Read the model definition and answer for the solid it produces. Units are mm, in the model's axes. Give positions to 0.01 mm unless a question says otherwise; leave off trailing zeros. Order: outer loops, then holes, each group sorted by start corner. A loop starts at its lowest first (then second) coordinate and runs counter-clockwise, first axis right, second up. Notation, with made-up numbers: (33.5, -35.5) -> (77.5, -35.5) arc R21 ccw to (77.5, -27.5) -> close; hole circle Ø10 at (30.25, -13). An arc over 180 degrees is marked (long way). Answer as CSV lines item,"result". Start each with the question number.
1) Straight lines are drawn through the part: L1, parallel to Y at x = 5.5, z = 0.6; L2, parallel to X at y = -6.5, z = 0.8; L3, parallel to Y at x = -12, z = -0.85. For each, find the intervals that lie inside material, in ascending order. Write a range as from..to.
2) Find section B-B (y = -24). Determine the outline of the cut face in (x, z), and give its area (3 significant figures).
3) Find section D-D (y = -3). Determine the outline of the cut face in (x, z), and give its area (3 significant figures).
4) Find section C-C (z = -1.1). State how many separate pieces and enclosed holes the cut face has, and give its area (3 significant figures).
5) Flat-ended cylindrical pins translate along their axes: pin 1 Ø1.5 at (x, z) = (18, 1) entering from -Y; pin 2 Ø6 at (x, y) = (-18.5, -17) entering from -Z. Find the tip coordinate at first contact, or state that the pin passes through.
6) Find section A-A (x = 3). Determine the outline of the cut face in (y, z).
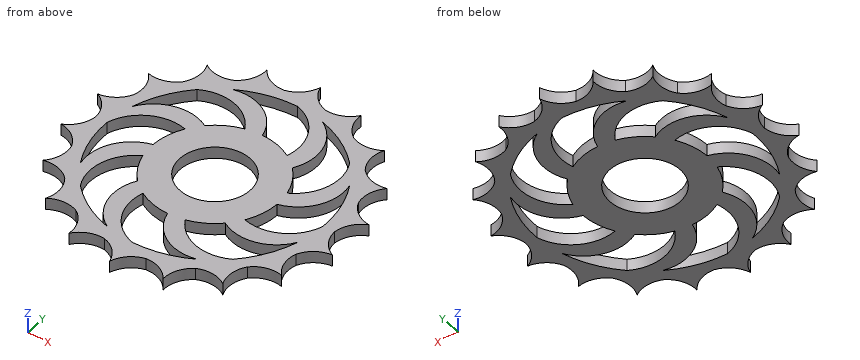
```python
from build123d import *

# Parameters (mm, degrees)
SALIENTE_EXTRUIR1_DEPTH = 1.5875
CROQUIS2_R              = 9.525
CORTAR_EXTRUIR1_DEPTH   = 4.175


with BuildPart() as part:
    # Croquis1 → Saliente-Extruir1 (new body, symmetric)
    with BuildSketch(Plane.XY):
        with BuildLine():
            ThreePointArc((0, 38.1), (-2.105039418, 34.526506764), (-5.733862827, 32.518352004))
            ThreePointArc((-5.733862827, 32.518352004), (-9.830670784, 33.164269511), (-13.030967461, 35.802288852))
            ThreePointArc((-13.030967461, 35.802288852), (-13.7868508, 31.724337744), (-16.51, 28.596158833))
            ThreePointArc((-16.51, 28.596158833), (-20.580657004, 27.801931903), (-24.490207929, 29.186293283))
            ThreePointArc((-24.490207929, 29.186293283), (-23.805764502, 25.09574539), (-25.294787512, 21.224846872))
            ThreePointArc((-25.294787512, 21.224846872), (-28.848312252, 19.086270994), (-32.995567884, 19.05))
            ThreePointArc((-32.995567884, 19.05), (-30.95335167, 15.440235769), (-31.028650338, 11.293505133))
            ThreePointArc((-31.028650338, 11.293505133), (-33.636435286, 8.06852412), (-37.52117539, 6.615995569))
            ThreePointArc((-37.52117539, 6.615995569), (-34.367507804, 3.922405841), (-33.02, 0))
            ThreePointArc((-33.02, 0), (-34.367507804, -3.922405841), (-37.52117539, -6.615995569))
            ThreePointArc((-37.52117539, -6.615995569), (-33.636435286, -8.06852412), (-31.028650338, -11.293505133))
            ThreePointArc((-31.028650338, -11.293505133), (-30.95335167, -15.440235769), (-32.995567884, -19.05))
            ThreePointArc((-32.995567884, -19.05), (-28.848312252, -19.086270994), (-25.294787512, -21.224846872))
            ThreePointArc((-25.294787512, -21.224846872), (-23.805764502, -25.09574539), (-24.490207929, -29.186293283))
            ThreePointArc((-24.490207929, -29.186293283), (-20.580657004, -27.801931903), (-16.51, -28.596158833))
            ThreePointArc((-16.51, -28.596158833), (-13.7868508, -31.724337744), (-13.030967461, -35.802288852))
            ThreePointArc((-13.030967461, -35.802288852), (-9.830670784, -33.164269511), (-5.733862827, -32.518352004))
            ThreePointArc((-5.733862827, -32.518352004), (-2.105039418, -34.526506764), (0, -38.1))
            ThreePointArc((0, -38.1), (2.105039418, -34.526506764), (5.733862827, -32.518352004))
            ThreePointArc((5.733862827, -32.518352004), (9.830670784, -33.164269511), (13.030967461, -35.802288852))
            ThreePointArc((13.030967461, -35.802288852), (13.7868508, -31.724337744), (16.51, -28.596158833))
            ThreePointArc((16.51, -28.596158833), (20.580657004, -27.801931903), (24.490207929, -29.186293283))
            ThreePointArc((24.490207929, -29.186293283), (23.805764502, -25.09574539), (25.294787512, -21.224846872))
            ThreePointArc((25.294787512, -21.224846872), (28.848312252, -19.086270994), (32.995567884, -19.05))
            ThreePointArc((32.995567884, -19.05), (30.95335167, -15.440235769), (31.028650338, -11.293505133))
            ThreePointArc((31.028650338, -11.293505133), (33.636435286, -8.06852412), (37.52117539, -6.615995569))
            ThreePointArc((37.52117539, -6.615995569), (34.367507804, -3.922405841), (33.02, 0))
            ThreePointArc((33.02, 0), (34.367507804, 3.922405841), (37.52117539, 6.615995569))
            ThreePointArc((37.52117539, 6.615995569), (33.636435286, 8.06852412), (31.028650338, 11.293505133))
            ThreePointArc((31.028650338, 11.293505133), (30.95335167, 15.440235769), (32.995567884, 19.05))
            ThreePointArc((32.995567884, 19.05), (28.848312252, 19.086270994), (25.294787512, 21.224846872))
            ThreePointArc((25.294787512, 21.224846872), (23.805764502, 25.09574539), (24.490207929, 29.186293283))
            ThreePointArc((24.490207929, 29.186293283), (20.580657004, 27.801931903), (16.51, 28.596158833))
            ThreePointArc((16.51, 28.596158833), (13.7868508, 31.724337744), (13.030967461, 35.802288852))
            ThreePointArc((13.030967461, 35.802288852), (9.830670784, 33.164269511), (5.733862827, 32.518352004))
            ThreePointArc((5.733862827, 32.518352004), (2.105039418, 34.526506764), (0, 38.1))
        make_face()
    extrude(amount=SALIENTE_EXTRUIR1_DEPTH, both=True)

    # Croquis2 → Cortar-Extruir1 (cut, through all)
    with BuildSketch(Plane.XY.offset(1.5875)):
        Circle(CROQUIS2_R)
        with BuildLine():
            ThreePointArc((8.5725, 14.848005548), (4.437452528, 16.560798292), (0, 17.145))
            ThreePointArc((0, 17.145), (-5.659104508, 24.58631503), (-14.9225, 25.846528176))
            ThreePointArc((-14.9225, 25.846528176), (-7.724454401, 28.828056286), (0, 29.845))
            ThreePointArc((0, 29.845), (7.392229248, 24.121925656), (8.5725, 14.848005548))
        make_face()
        with BuildLine():
            ThreePointArc((21.103601885, 21.103601885), (14.9225, 25.846528176), (7.724454401, 28.828056286))
            ThreePointArc((7.724454401, 28.828056286), (13.383558909, 21.386741255), (12.123345763, 12.123345763))
            ThreePointArc((12.123345763, 12.123345763), (14.848005548, 8.5725), (16.560798292, 4.437452528))
            ThreePointArc((16.560798292, 4.437452528), (22.283872636, 11.829681777), (21.103601885, 21.103601885))
        make_face()
        with BuildLine():
            ThreePointArc((29.845, 0), (28.828056286, 7.724454401), (25.846528176, 14.9225))
            ThreePointArc((25.846528176, 14.9225), (24.58631503, 5.659104508), (17.145, 0))
            ThreePointArc((17.145, 0), (16.560798292, -4.437452528), (14.848005548, -8.5725))
            ThreePointArc((14.848005548, -8.5725), (24.121925656, -7.392229248), (29.845, 0))
        make_face()
        with BuildLine():
            ThreePointArc((21.103601885, -21.103601885), (25.846528176, -14.9225), (28.828056286, -7.724454401))
            ThreePointArc((28.828056286, -7.724454401), (21.386741255, -13.383558909), (12.123345763, -12.123345763))
            ThreePointArc((12.123345763, -12.123345763), (8.5725, -14.848005548), (4.437452528, -16.560798292))
            ThreePointArc((4.437452528, -16.560798292), (11.829681777, -22.283872636), (21.103601885, -21.103601885))
        make_face()
        with BuildLine():
            ThreePointArc((0, -29.845), (7.724454401, -28.828056286), (14.9225, -25.846528176))
            ThreePointArc((14.9225, -25.846528176), (5.659104508, -24.58631503), (0, -17.145))
            ThreePointArc((0, -17.145), (-4.437452528, -16.560798292), (-8.5725, -14.848005548))
            ThreePointArc((-8.5725, -14.848005548), (-7.392229248, -24.121925656), (0, -29.845))
        make_face()
        with BuildLine():
            ThreePointArc((-21.103601885, -21.103601885), (-14.9225, -25.846528176), (-7.724454401, -28.828056286))
            ThreePointArc((-7.724454401, -28.828056286), (-13.383558909, -21.386741255), (-12.123345763, -12.123345763))
            ThreePointArc((-12.123345763, -12.123345763), (-14.848005548, -8.5725), (-16.560798292, -4.437452528))
            ThreePointArc((-16.560798292, -4.437452528), (-22.283872636, -11.829681777), (-21.103601885, -21.103601885))
        make_face()
        with BuildLine():
            ThreePointArc((-29.845, 0), (-28.828056286, -7.724454401), (-25.846528176, -14.9225))
            ThreePointArc((-25.846528176, -14.9225), (-24.58631503, -5.659104508), (-17.145, 0))
            ThreePointArc((-17.145, 0), (-16.560798292, 4.437452528), (-14.848005548, 8.5725))
            ThreePointArc((-14.848005548, 8.5725), (-24.121925656, 7.392229248), (-29.845, 0))
        make_face()
        with BuildLine():
            ThreePointArc((-21.103601885, 21.103601885), (-25.846528176, 14.9225), (-28.828056286, 7.724454401))
            ThreePointArc((-28.828056286, 7.724454401), (-21.386741255, 13.383558909), (-12.123345763, 12.123345763))
            ThreePointArc((-12.123345763, 12.123345763), (-8.5725, 14.848005548), (-4.437452528, 16.560798292))
            ThreePointArc((-4.437452528, 16.560798292), (-11.829681777, 22.283872636), (-21.103601885, 21.103601885))
        make_face()
    extrude(amount=-CORTAR_EXTRUIR1_DEPTH, mode=Mode.SUBTRACT)


solid = part.part
```
Findings below:
1,L1,"-32.58..-29.33, -24.49..-18.12, -16.24..-7.78, 7.78..16.24, 26.62..32.58"
1,L2,"-37.29..-29.13, -25.03..-19.23, -15.87..-6.96, 6.96..15.87, 25.47..37.29"
1,L3,"-34.61..-27.33, -24.64..12.25, 22.33..26.25, 27.33..34.61"
2,outline,"(-24, -1.59) -> (-17.74, -1.59) -> (-17.74, 1.59) -> (-24, 1.59) -> close; (-12.36, -1.59) -> (-7.46, -1.59) -> (-7.46, 1.59) -> (-12.36, 1.59) -> close; (4.75, -1.59) -> (24, -1.59) -> (24, 1.59) -> (4.75, 1.59) -> close"
2,area,"96.5 mm²"
3,outline,"(-33.83, -1.59) -> (-29.69, -1.59) -> (-29.69, 1.59) -> (-33.83, 1.59) -> close; (-22.49, -1.59) -> (-9.04, -1.59) -> (-9.04, 1.59) -> (-22.49, 1.59) -> close; (9.04, -1.59) -> (16.88, -1.59) -> (16.88, 1.59) -> (9.04, 1.59) -> close; (28.58, -1.59) -> (33.83, -1.59) -> (33.83, 1.59) -> (28.58, 1.59) -> close"
3,area,"97.4 mm²"
4,separate pieces,"1"
4,enclosed holes,"9"
4,area,"2,180 mm²"
5,pin 1,"y = -28.28"
5,pin 2,"through"
6,outline,"(-33.78, -1.59) -> (-29.69, -1.59) -> (-29.69, 1.59) -> (-33.78, 1.59) -> close; (-22.49, -1.59) -> (-9.04, -1.59) -> (-9.04, 1.59) -> (-22.49, 1.59) -> close; (9.04, -1.59) -> (16.88, -1.59) -> (16.88, 1.59) -> (9.04, 1.59) -> close; (28.58, -1.59) -> (33.78, -1.59) -> (33.78, 1.59) -> (28.58, 1.59) -> close"
